Check sheet for the drawn part. Datum: minimum x, y, z corner. Units: mm. A direction names the side the tool comes from. Give positions to 0.01 mm unless a question says otherwise; leave off trailing zeros. Write each loop counter-clockwise with the first axis right and the second up, starting at its lowest first coordinate (ties: lowest second). Pieces come first, ordered by that corner, then holes. Notation, with made-up numbers: (31, -21) - (78, -21) arc R30 cw to (78, 1) - close; hole circle Ø8 at (-12.5, 45). An arc over 180 degrees is marked (long way). Use a Markdown table: item, result.
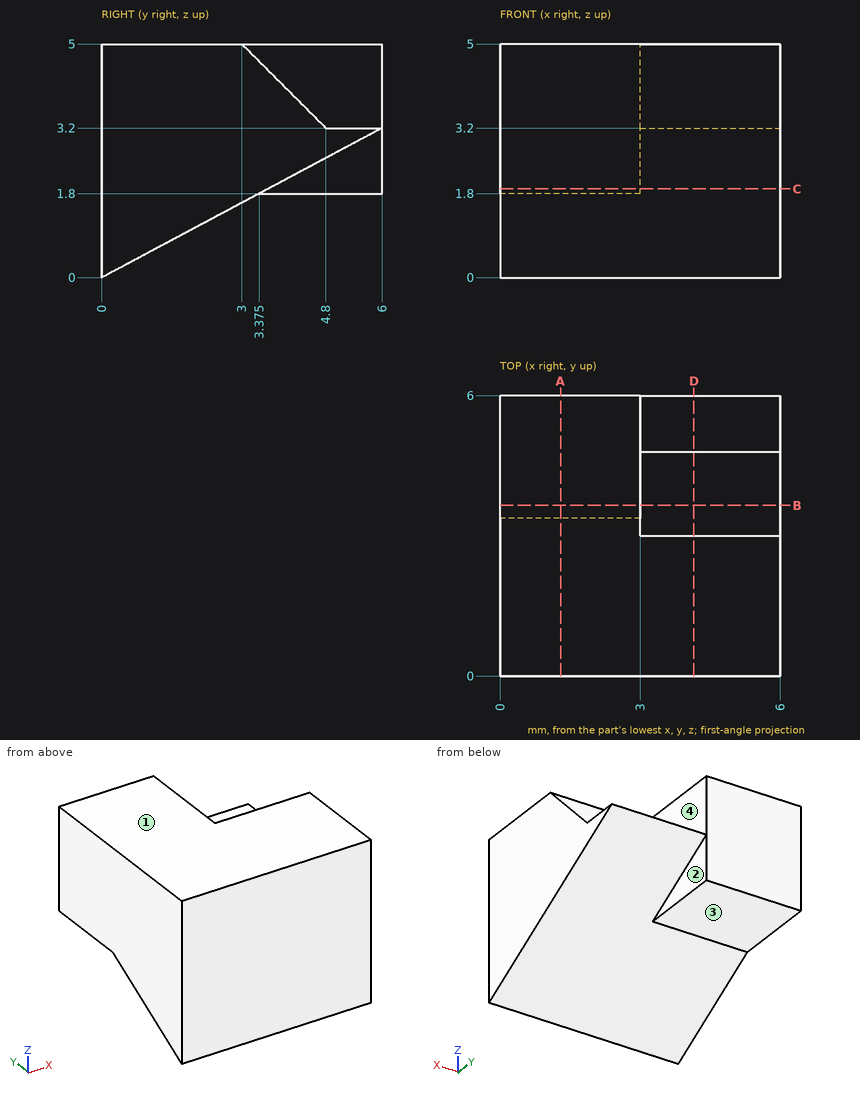
1) Section check D-D on x = 4.15. Record the boundary of the cut face in (y, z), then the cut area to 3 significant figures.
Working result:
| item | result |
|---|---|
| outline | (0, 0) - (6, 3.2) - (4.8, 3.2) - (3, 5) - (0, 5) - close |
| area | 16.6 mm² |
2) Depth check by flat-ended pin: P1, Ø2, axis at x = 4, y = 4, coming from the -Z side; P2, Ø1.3, axis at x = 4.5, y = 5.5, coming from the +Z side; P3, Ø0.5, axis at y = 4.5, z = 4, coming from the +X side. Enter the tip coordinate at first touch or a pass-through.
Working result:
| item | result |
|---|---|
| P1 | stops at z = 1.6 |
| P2 | stops at z = 3.2 |
| P3 | stops at x = 3 |
3) Section check C-C on z = 1.9. Record the boundary of the cut face in (x, y).
Working result:
| item | result |
|---|---|
| outline | (0, 0) - (6, 0) - (6, 3.56) - (3, 3.56) - (3, 6) - (0, 6) - close |
4) Section check A-A on x = 1.3. Record the boundary of the cut face in (y, z) (3 decimals), then the cut area to 3 significant figures.
Working result:
| item | result |
|---|---|
| outline | (0, 0) - (3.375, 1.8) - (6, 1.8) - (6, 5) - (0, 5) - close |
| area | 22.2 mm² |
5) Section check B-B on y = 3.65. Record the boundary of the cut face in (x, z), then the cut area to 3 significant figures.
Working result:
| item | result |
|---|---|
| outline | (0, 1.8) - (3, 1.8) - (3, 1.95) - (6, 1.95) - (6, 4.35) - (3, 4.35) - (3, 5) - (0, 5) - close |
| area | 16.8 mm² |
6) Set-up check for the marked faces 1, 2, 3 and 4: record each of +Z, -Z, +X, -X, +Y, -Y from which the full face is reachable in a straight line by a thin tool's end or side.
Working result:
| item | result |
|---|---|
| face 1 | +Z, +X, -X, +Y, -Y |
| face 2 | -Z, +X, +Y |
| face 3 | -Z, +X, -X, +Y |
| face 4 | +Z, +X, +Y |
7) Material ranges on L1, parallel to Z at x = 0.35, y = 5.2; L2, parallel to X at y = 5.35, z = 2.35; L3, parallel to Y at x = 3.15, z = 2.55, recorded low to high. Write a range as from..to.
Working result:
| item | result |
|---|---|
| L1 | z = 1.8..5 |
| L2 | x = 0..3 |
| L3 | y = 0..4.78 |
